```python
from build123d import *

# Parameters (mm, degrees)
SKETCH1_R           = 5
BOSS_EXTRUDE1_DEPTH = 200
SKETCH3_R           = 5
SKETCH3_R_2         = 4
CUT_EXTRUDE1_DEPTH  = 10
CUT_EXTRUDE2_START  = -10
SKETCH4_R           = 5
SKETCH4_R_2         = 4
CUT_EXTRUDE2_DEPTH  = 10
SKETCH5_W           = 1.5
SKETCH5_H           = 10
BOSS_EXTRUDE2_DEPTH = 50
SKETCH6_R           = 2.5
CUT_EXTRUDE3_DEPTH  = 50
FILLET1_R           = 4
SKETCH8_R           = 4
BOSS_EXTRUDE3_DEPTH = 40


with BuildPart() as part:
    # Sketch1 → Boss-Extrude1 (new body)
    with BuildSketch(Plane(origin=(0, 0, 0), x_dir=(0, 0, -1), z_dir=(1, 0, 0))):
        Circle(SKETCH1_R)
    extrude(amount=BOSS_EXTRUDE1_DEPTH)

    # Sketch3 → Cut-Extrude1 (cut)
    with BuildSketch(Plane.ZY):
        Circle(SKETCH3_R)
        Circle(SKETCH3_R_2, mode=Mode.SUBTRACT)
    extrude(amount=-CUT_EXTRUDE1_DEPTH, mode=Mode.SUBTRACT)

    # Sketch4 → Cut-Extrude2 (cut)
    with BuildSketch(Plane(origin=(200, 0, 0), x_dir=(0, 0, -1), z_dir=(1, 0, 0)).offset(CUT_EXTRUDE2_START)):
        with Locations(Location((0, 0, 0), (0, 0, 180))):
            Circle(SKETCH4_R)
        with Locations(Location((0, 0, 0), (0, 0, 180))):
            Circle(SKETCH4_R_2, mode=Mode.SUBTRACT)
    extrude(amount=CUT_EXTRUDE2_DEPTH, mode=Mode.SUBTRACT)

    # Sketch5 → Boss-Extrude2 (add)
    with BuildSketch(Plane(origin=(0, 0, 0), x_dir=(1, 0, 0), z_dir=(0, 1, 0))):
        with Locations((24.122206293, 0)):
            Rectangle(SKETCH5_W, SKETCH5_H)
    extrude(amount=BOSS_EXTRUDE2_DEPTH)

    # Sketch6 → Cut-Extrude3 (cut)
    with BuildSketch(Plane.ZY.offset(-23.372206293)):
        with Locations((0, 45)):
            Circle(SKETCH6_R)
    extrude(amount=-CUT_EXTRUDE3_DEPTH, mode=Mode.SUBTRACT)

    # Fillet1
    fillet1_edges = [part.edges().sort_by_distance(p)[0] for p in [
        (24.122206293, 50, -5),
        (24.122206293, 50, 5),
    ]]
    fillet(fillet1_edges, radius=FILLET1_R)

    # Sketch8 → Boss-Extrude3 (add)
    with BuildSketch(Plane(origin=(0, 0, 0), x_dir=(0, 0.7071067811865462, 0.7071067811865488), z_dir=(-8.296615423026079e-08, 0.7071067811865465, -0.7071067811865439))):
        with Locations((0, 155)):
            Circle(SKETCH8_R)
        with Locations((0, 85)):
            Circle(SKETCH8_R)
    extrude(amount=-BOSS_EXTRUDE3_DEPTH)


solid = part.part
```
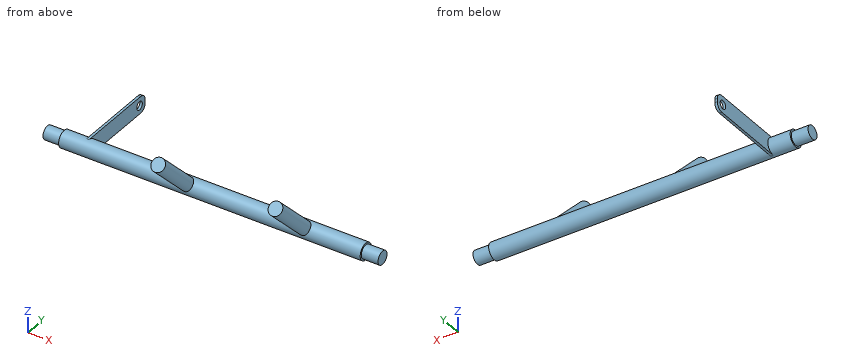
Design review of the part built by this model. Coordinates are the model's own, in mm. Round coordinates to 2 decimals unless told otherwise and drop trailing zeros. Write each loop counter-clockwise with the first axis right and the second up, starting at its lowest first coordinate (ties: lowest second). Pieces come first, ordered by that corner, then holes.
Item 1: We need section A-A on x = 21. Write out the cut boundary in (y, z), and give its area (3 significant figures).
Item 2: Clearance check with flat-ended pins moving along their axes: pin 1 Ø8 at (y, z) = (-19.5, 23.5) entering from +X; pin 2 Ø2 at (y, z) = (34.5, 2) entering from +X; pin 3 Ø11 at (y, z) = (33, 1) entering from -X. State where each tip first meets the part, or that it passes through.
Item 3: For probe 1 along Y at (x, z) = (24.55, 0); probe 2 along X at (y, z) = (19, -2.5); probe 3 along Y at (x, z) = (23, 0), list the stretches that pass through material, from the lowest coordinate up.
Returned:
1. outline: circle Ø10 at (0, 0)
1. area: 78.5 mm2
2. pin 1: stops at x = 159
2. pin 2: stops at x = 24.87
2. pin 3: stops at x = 23.37
3. probe 1: y = -5 to 42.5, 47.5 to 50
3. probe 2: x = 23.37 to 24.87
3. probe 3: y = -5 to 5
